Geometry: final body of the model. Coordinates: model frame, mm. A direction names the side the tool comes from. Round coordinates to 2 decimals unless told otherwise and drop trailing zeros. Write each loop counter-clockwise with the first axis right and the second up, starting at its lowest first coordinate (ties: lowest second). Pieces come first, ordered by that corner, then holes. Notation, with made-up numbers: (-24.5, 57) -> (-1.5, 57) arc R30 cw to (-1.5, 91) -> close; hole circle Ø10 at (-36, -37). An arc over 180 degrees is marked (long way). Use one line per item in the form item = value. Start each with the question number.
1. Cut plane D-D, the plane x = 0. Return the cut outline in (y, z), plus the area to 3 significant figures.
2. Cut plane A-A, the plane y = -2.5. Return the cut outline in (x, z), plus the area to 3 significant figures.
3. Line query: L1, parallel to X at y = -14.75, z = -9.5; L2, parallel to X at y = -19.75, z = -26.5; L3, parallel to Z at x = -2.5, y = -21.25. Output: solid intervals per line, ascending.
4. Reachability of faces 1 (the face through (-9.275, -12, -43)), 2 (the face through (-42, -12, -5)), 3 (the face through (42, -12, -5)) from +Z, -Z, +X, -X, +Y, -Y: full face, straight path, thin tool, end or side. Return the list, or none.
5. Draft query along X for faces 4 (the face through (9.222, -12, -42)), 5 (the face through (-14.275, -12, -41)), 6 (the face through (15.18, -12.32, -36.01)). Return one class per face: pulls with the +X half, pulls with the -X half, needs draft (parallel to the pull), parting line crosses it, or undercut.
6. Cut plane C-C, the plane z = -13.5. Return the cut outline in (x, y).
7. Cut plane B-B, the plane z = -26. Return the cut outline in (x, y), plus the area to 3 significant figures.
8. Pin query (flat end, axial travel): pin 1 Ø1.6 at (y, z) = (-12.5, -42) entering from -X; pin 2 Ø6 at (x, y) = (31.5, -17.5) entering from -Z; pin 3 Ø1 at (y, z) = (-10, -42) entering from +X. Return the tip coordinate at first contact, or that it passes through.
```python
from build123d import *

# Parameters (mm, degrees)
F1_DEPTH    = 25
F2_T1_DEPTH = 25


# Not quite as in the source:
# - a fillet or chamfer that OpenCascade refuses, or shapes differently, is made with other operations: its cross-section is extruded or revolved along the edge and cut away or added


with BuildPart() as f1:
    # F0 (on Front) → F1 (new body)
    with BuildSketch(Plane.XZ):
        with BuildLine():
            ThreePointArc((36, 0), (0, -36), (-36, 0))
            Line((-36, 0), (-38.5, 0))
            Line((-38.5, 0), (-46, 0))
            Line((-46, 0), (-46, -5))
            Line((-46, -5), (-38.1739439933, -5))
            ThreePointArc((-38.1739439933, -5), (-26.2977937101, -28.1189623916), (-2.4365316343, -38.4228228218))
            Line((-2.4365316343, -38.4228228218), (-14.2752447595, -38.6175373625))
            Line((-14.2752447595, -38.6175373625), (-14.2752447595, -43.6175822914))
            Line((-14.2752447595, -43.6175822914), (-9.2752447595, -43.5353459289))
            Line((-9.2752447595, -43.5353459289), (-9.2752447595, -41.5353459289))
            Line((-9.2752447595, -41.5353459289), (9.222253505, -41.2311125346))
            Line((9.222253505, -41.2311125346), (9.222253505, -43.2311125346))
            Line((9.222253505, -43.2311125346), (14.222253505, -43.1488761722))
            Line((14.222253505, -43.1488761722), (14.222253505, -38.1488312433))
            Line((14.222253505, -38.1488312433), (3.6987732294, -38.3219137909))
            ThreePointArc((3.6987732294, -38.3219137909), (26.7566551829, -27.682691405), (38.1739439933, -5))
            Line((38.1739439933, -5), (46, -5))
            Line((46, -5), (46, 0))
            Line((46, 0), (38.5, 0))
            Line((38.5, 0), (36, 0))
        make_face()
    extrude(amount=F1_DEPTH)

    # F2: fillet of radius 5 on 2 edges, made by hand

    # F2_s2 → F2_t1 (join)
    with BuildSketch(Plane.XZ):
        with BuildLine():
            ThreePointArc((-14.2752447595, -38.6175373625), (-15.118767178, -36.2023611517), (-17.0464798519, -34.5205377226))
            ThreePointArc((-17.0464798519, -34.5205377226), (-9.9349832104, -37.1960496371), (-2.4365316343, -38.4228228218))
            Line((-2.4365316343, -38.4228228218), (-14.2752447595, -38.6175373625))
        make_face()
        with BuildLine():
            ThreePointArc((16.9380433228, -34.5738729158), (15.1563460299, -36.0394019773), (14.222253505, -38.1488312433))
            Line((14.222253505, -38.1488312433), (3.6987732294, -38.3219137909))
            ThreePointArc((3.6987732294, -38.3219137909), (10.4872065848, -37.0441425606), (16.9380433228, -34.5738729158))
        make_face()
    extrude(amount=F2_T1_DEPTH)


solid = f1.part
```
Outcome:
q1.outline = (-25, -41.38) -> (0, -41.38) -> (0, -36) -> (-25, -36) -> close
q1.area = 135 mm^2
q2.outline = (-46, -5) -> (-38.17, -5) arc R38.5 ccw to (-17.05, -34.52) arc R5 cw to (-14.28, -38.62) -> (-14.28, -43.62) -> (-9.28, -43.54) -> (-9.28, -41.54) -> (9.22, -41.23) -> (9.22, -43.23) -> (14.22, -43.15) -> (14.22, -38.15) arc R5 cw to (16.94, -34.57) arc R38.5 ccw to (38.17, -5) -> (46, -5) -> (46, 0) -> (36, 0) arc R36 cw to (-36, 0) -> (-46, 0) -> close
q2.area = 500 mm^2
q3.L1 = -37.31 to -34.72, 34.72 to 37.31
q3.L2 = -27.93 to -24.37, 24.37 to 27.93
q3.L3 = -41.42 to -35.91
q4.face_1 = -Z, +Y, -Y
q4.face_2 = -Z, -X, +Y, -Y
q4.face_3 = -Z, +X, +Y, -Y
q5.face_4 = undercut
q5.face_5 = pulls with the -X half
q5.face_6 = pulls with the +X half
q6.outline = (-36.06, -25) -> (-33.37, -25) -> (-33.37, 0) -> (-36.06, 0) -> close; (33.37, -25) -> (36.06, -25) -> (36.06, 0) -> (33.37, 0) -> close
q7.outline = (-28.39, -25) -> (-24.9, -25) -> (-24.9, 0) -> (-28.39, 0) -> close; (24.9, -25) -> (28.39, -25) -> (28.39, 0) -> (24.9, 0) -> close
q7.area = 175 mm^2
q8.pin_1 = -14.28
q8.pin_2 = -25.88
q8.pin_3 = 14.22
